Read the model definition and answer for the solid it produces. Units are mm, in the model's axes. Face numbers are marked on the shaded views. A direction names the side the tool comes from. Coordinates: 2 decimals unless noted, no trailing zeros. Write each loop counter-clockwise with the first axis right and the second up, starting at its lowest first coordinate (ties: lowest second). Pieces come first, ordered by that corner, then holes. Notation, with made-up numbers: M -7,62 L 7,62 A29 ccw 7,95 Z; hole C 8.5,83.5 d2. An arc over 180 degrees is marked long. Write item = value, one per line.
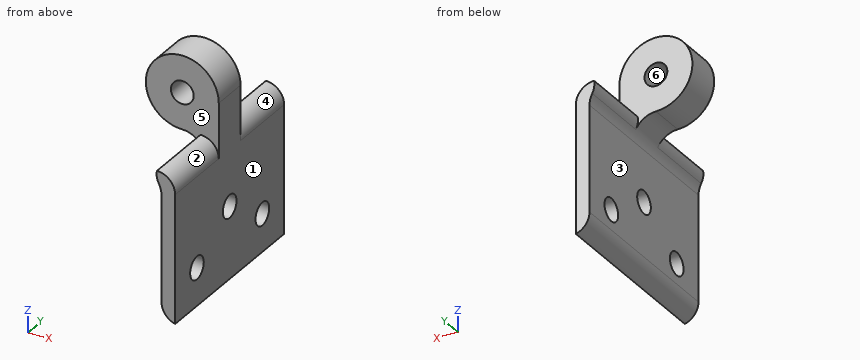
from build123d import *

# Parameters (mm, degrees)
SKETCH1_R               = 1.25
BOSS_EXTRUDE1_DEPTH     = 20
CUT_EXTRUDE1_DEPTH      = 30.021543722
CUT_EXTRUDE1_DEPTH_BACK = 30.021543722
SKETCH2_R               = 1.25
CUT_EXTRUDE3_DEPTH      = 29.565713714
CUT_EXTRUDE3_DEPTH_BACK = 29.565713714
SKETCH3_W               = 10
SKETCH3_H               = 8
SKETCH3_W_2             = 9.357078711
FILLET3_R               = 2
FILLET4_R               = 2
FILLET8_R               = 2
FILLET9_R               = 2
FILLET11_R              = 2


with BuildPart() as part:
    # Sketch1 → Boss-Extrude1 (new body)
    with BuildSketch(Plane(origin=(0, 0, 0), x_dir=(1, 0, 0), z_dir=(0, 1, 0))):
        with BuildLine():
            Line((4, 0), (4, 20))
            Line((4, 20), (2.5, 20))
            Line((2.5, 20), (2.5, 15.120027663))
            Line((2.5, 15.120027663), (2.5, 6.5))
            ThreePointArc((2.5, 6.5), (1.767766953, 4.732233047), (0, 4))
            ThreePointArc((0, 4), (-2.828427125, -2.828427125), (4, 0))
        make_face()
        with Locations(Location((0, 0, 0), (0, 0, 270))):
            Circle(SKETCH1_R, mode=Mode.SUBTRACT)
    extrude(amount=BOSS_EXTRUDE1_DEPTH)

    # Sketch2 → Cut-Extrude1 (cut, two sides: drawn at the far end of the back side and taken through both)
    with BuildSketch(Plane.ZY.offset(-2.5).offset(-CUT_EXTRUDE1_DEPTH_BACK)):
        with Locations((-12.139236455, 10)):
            Circle(SKETCH2_R)
        with Locations((-15.86873762, 4)):
            Circle(SKETCH2_R)
        with Locations((-15.86873762, 16)):
            Circle(SKETCH2_R)
    extrude(amount=CUT_EXTRUDE1_DEPTH + CUT_EXTRUDE1_DEPTH_BACK, mode=Mode.SUBTRACT)

    # Sketch3 → Cut-Extrude3 (cut, two sides: drawn at the far end of the back side and taken through both)
    with BuildSketch(Plane(origin=(0, 0, 0), x_dir=(0, 0, -1), z_dir=(1, 0, 0)).offset(-CUT_EXTRUDE3_DEPTH_BACK)):
        with Locations((-1, 4)):
            Rectangle(SKETCH3_W, SKETCH3_H)
        with Locations((-0.678539356, 16)):
            Rectangle(SKETCH3_W_2, SKETCH3_H)
    extrude(amount=CUT_EXTRUDE3_DEPTH + CUT_EXTRUDE3_DEPTH_BACK, mode=Mode.SUBTRACT)

    # Fillet3
    fillet3_edges = [part.edges().sort_by_distance(p)[0] for p in [
        (4, 16, -4),
    ]]
    fillet(fillet3_edges, radius=FILLET3_R)

    # Fillet4
    # the kernel refuses this fillet: 2 mm, written as the material it takes off along each edge
    with BuildSketch(Plane(origin=(0, 12, -4), x_dir=(0.8581589387978472, 0, -0.513384101586086), z_dir=(0, 1, 0))) as fillet4_piece_1:
        with BuildLine():
            CenterArc((3.593688711, -1.716317878), FILLET4_R, 120.889507128, 38.942441269)
            Line((1.716317878, -1.026768203), (0, 0))
            ThreePointArc((0, 0), (1.283460254, -0.354602653), (2.566920508, 0))
        make_face()
    extrude(amount=14.41730127, mode=Mode.SUBTRACT)

    # Fillet8
    fillet8_edges = [part.edges().sort_by_distance(p)[0] for p in [
        (4, 4, -4),
    ]]
    fillet(fillet8_edges, radius=FILLET8_R)

    # Fillet9
    # the kernel refuses this fillet: 2 mm, written as the material it takes off along each edge
    with BuildSketch(Plane(origin=(0, -6.41730127, -4), x_dir=(0.8581589387978472, 0, -0.513384101586086), z_dir=(0, 1, 0))) as fillet9_piece_1:
        with BuildLine():
            CenterArc((3.593688711, -1.716317878), FILLET9_R, 120.889507128, 38.942441269)
            Line((1.716317878, -1.026768203), (1.678770461, -1.01297721))
            ThreePointArc((1.678770461, -1.01297721), (0.837623575, -0.547710459), (-0.020535364, -0.034326358))
            Line((-0.020535364, -0.034326358), (0.020535364, 0.034326358))
            ThreePointArc((0.020535364, 0.034326358), (1.283460254, -0.314602653), (2.546385144, 0.034326358))
            Line((2.546385144, 0.034326358), (2.566920508, 0))
        make_face()
    extrude(amount=14.41730127, mode=Mode.SUBTRACT)

    # Fillet11
    # the kernel refuses this fillet: 2 mm, written as the material it takes off along each edge
    with BuildSketch(Plane(origin=(2.5, -4.841229183, -20), x_dir=(1, 0, 0), z_dir=(0, 1, 0))) as fillet11_piece_1:
        with BuildLine():
            CenterArc((2, -1.936491673), FILLET11_R, 104.477512186, 75.522487814)
            Line((0, -1.936491673), (-0.04, -1.936491673))
            Line((-0.04, -1.936491673), (-0.04, 0))
            Line((-0.04, 0), (0, 0.04))
            ThreePointArc((0, 0.04), (0.75, 0.04), (1.49, 0.038729833))
            Line((1.49, 0.038729833), (1.5, 0))
        make_face()
    extrude(amount=29.682458366, mode=Mode.SUBTRACT)


solid = part.part
Item 1: Find section D-D (z = -10). Determine the outline of the cut face in (x, y).
Worked answers:
outline = M 2.5,0 L 4,0 L 4,20 L 2.5,20 Z
Item 2: Find section B-B (y = 16). Determine the outline of the cut face in (x, z), and give its area (3 significant figures).
Worked answers:
outline = M 2,-4 A2 ccw 2.2,-5.32 A2.5 cw 2.5,-6.5 L 2.5,-14.62 L 4,-14.62 L 4,-6 A2 ccw Z; M 2.5,-18.06 A2 ccw 4,-20 L 4,-17.12 L 2.5,-17.12 Z
area = 19.4 mm²
Item 3: For a pull along X with two mould halves and no side action, classify the marked faces 3, 4, 5 and 6 as released by +X, released by -X, zero draft, split by the parting line, or undercut.
Worked answers:
face_3 = released by -X
face_4 = released by +X
face_5 = zero draft
face_6 = undercut
Item 4: Find section A-A (y = 10). Determine the outline of the cut face in (x, z), and give its area (3 significant figures).
Worked answers:
outline = M 0,-4 A2.5 cw 2.5,-6.5 L 2.5,-10.89 L 4,-10.89 L 4,0 A4 ccw long Z; M 2.5,-18.06 A2 ccw 4,-20 L 4,-13.39 L 2.5,-13.39 Z; hole C 0,0 d2.5
area = 69.6 mm²
Item 5: Consider line 1 along Y through (x, z) = (2.75, -0.75); line 2 along X through (y, z) = (16.25, -12.5); line 3 along X through (y, z) = (11.25, -0.75). Determine where each line is inside the solid, lowest interval first. Write a range as from..to.
Worked answers:
line_1 = 8..12
line_2 = 2.5..4
line_3 = -3.93..-1, 1..4
Item 6: Which of the six approach directions +Z, -Z, +X, -X, +Y, -Y give full straight-line access (tool end or side, diameter ignored) to the marked faces 1 and 2?
Worked answers:
face_1 = +Z, -Z, +X, +Y, -Y
face_2 = +Z, +X, -Y
Item 7: Find section C-C (x = 0.5). Determine the outline of the cut face in (y, z).
Worked answers:
outline = M 8,-4.05 L 12,-4.05 L 12,-1.15 L 8,-1.15 Z; M 8,1.15 L 12,1.15 L 12,3.97 L 8,3.97 Z
Item 8: Flat-ended cylindrical pins translate along their axes: pin 1 (3 mm diameter, centred on x = 0, z = 0, fed in from +Y); pin 2 (6 mm diameter, centred on y = 8, z = -15, fed in from -X); pin 3 (2 mm diameter, centred on y = 10, z = -12.14, fed in from -X); pin 4 (3 mm diameter, centred on y = 13, z = -0.5, fed in from +X). Find the tip coordinate at first contact, or state that the pin passes through.
Worked answers:
pin_1 = 12
pin_2 = 2.5
pin_3 = through
pin_4 = 4
